```python
from build123d import *

# Parameters (mm, degrees)
SKETCH_1_R             = 11
EXTRUDE_1_DEPTH        = 32
HOLE_WIZARD_M2_1_D     = 1.6
HOLE_WIZARD_M2_1_DEPTH = 5.2
HOLE_WIZARD_M2_1_TIP   = 0.480688495
CUT_EXTRUDE_START      = -3
SKETCH_5_R             = 11.838448527
SKETCH_5_R_2           = 10.75
CUT_EXTRUDE_1_DEPTH    = 0.05
CUT_EXTRUDE_START_2    = -30
SKETCH_5_2_R           = 11.838448527
SKETCH_5_2_R_2         = 10.75
CUT_EXTRUDE_2_DEPTH    = 0.05
SKETCH_6_R             = 12
EXTRUDE_2_DEPTH        = 13
SKETCH_7_R             = 5
EXTRUDE_3_DEPTH        = 3
SKETCH_8_R             = 3
EXTRUDE_4_DEPTH        = 4
SKETCH_9_R             = 1.5
EXTRUDE_5_DEPTH        = 13
SKETCH_10_W            = 5.142844332
SKETCH_10_H            = 1.571012966
CUT_EXTRUDE_3_DEPTH    = 8
HOLE_WIZARD_M2_2_D     = 1.6
HOLE_WIZARD_M2_2_DEPTH = 5.2
HOLE_WIZARD_M2_2_TIP   = 0.480688495


with BuildPart() as part:
    # Sketch 1 → Extrude 1 (new body)
    with BuildSketch(Plane.XY):
        Circle(SKETCH_1_R)
    extrude(amount=EXTRUDE_1_DEPTH)

    # Hole Wizard M2 _1
    with Locations(Plane(origin=(0, 8.5, 32), x_dir=(1, 0, 0), z_dir=(0, 0, 1))):
        with Locations((0, 0), (0, -17)):
            Hole(HOLE_WIZARD_M2_1_D / 2, depth=HOLE_WIZARD_M2_1_DEPTH)
            with Locations((0, 0, -(HOLE_WIZARD_M2_1_DEPTH + HOLE_WIZARD_M2_1_TIP / 2))):  # 118° drill point
                Cone(0, HOLE_WIZARD_M2_1_D / 2, HOLE_WIZARD_M2_1_TIP, mode=Mode.SUBTRACT)

    # Sketch 5 → Cut-Extrude 1 (cut)
    with BuildSketch(Plane(origin=(0, 0, 0), x_dir=(-1, 0, 0), z_dir=(0, 0, -1)).offset(CUT_EXTRUDE_START)):
        Circle(SKETCH_5_R)
        Circle(SKETCH_5_R_2, mode=Mode.SUBTRACT)
    extrude(amount=-CUT_EXTRUDE_1_DEPTH, mode=Mode.SUBTRACT)

    # Sketch 5_2 → Cut-Extrude 2 (cut)
    with BuildSketch(Plane(origin=(0, 0, 0), x_dir=(-1, 0, 0), z_dir=(0, 0, -1)).offset(CUT_EXTRUDE_START_2)):
        Circle(SKETCH_5_2_R)
        Circle(SKETCH_5_2_R_2, mode=Mode.SUBTRACT)
    extrude(amount=-CUT_EXTRUDE_2_DEPTH, mode=Mode.SUBTRACT)

    # Sketch 6 → Extrude 2 (add)
    with BuildSketch(Plane.XY.offset(32)):
        with Locations(Location((0, 0, 0), (0, 0, 180))):
            Circle(SKETCH_6_R)
    extrude(amount=EXTRUDE_2_DEPTH)

    # Sketch 7 → Extrude 3 (add)
    with BuildSketch(Plane.XY.offset(45)):
        Circle(SKETCH_7_R)
    extrude(amount=EXTRUDE_3_DEPTH)

    # Sketch 8 → Extrude 4 (add)
    with BuildSketch(Plane.XY.offset(45)):
        Circle(SKETCH_8_R)
    extrude(amount=EXTRUDE_4_DEPTH)

    # Sketch 9 → Extrude 5 (add)
    with BuildSketch(Plane.XY.offset(45)):
        with Locations(Location((0, 0, 0), (0, 0, 180))):
            Circle(SKETCH_9_R)
    extrude(amount=EXTRUDE_5_DEPTH)

    # Sketch 10 → Cut-Extrude 3 (cut)
    with BuildSketch(Plane.XY.offset(58)):
        with Locations((0.334320666, 1.635506483)):
            Rectangle(SKETCH_10_W, SKETCH_10_H)
    extrude(amount=-CUT_EXTRUDE_3_DEPTH, mode=Mode.SUBTRACT)

    # Hole Wizard M2 _2
    with Locations(Plane(origin=(0, 9.8, 45), x_dir=(1, 0, 0), z_dir=(0, 0, 1))):
        with Locations((0, 0), (8.487048957, -14.7), (-8.487048957, -14.7)):
            Hole(HOLE_WIZARD_M2_2_D / 2, depth=HOLE_WIZARD_M2_2_DEPTH)
            with Locations((0, 0, -(HOLE_WIZARD_M2_2_DEPTH + HOLE_WIZARD_M2_2_TIP / 2))):  # 118° drill point
                Cone(0, HOLE_WIZARD_M2_2_D / 2, HOLE_WIZARD_M2_2_TIP, mode=Mode.SUBTRACT)


solid = part.part
```
Geometry check sheet. Reference: the model listing, model coordinates, mm. A direction names the side the tool comes from. Coordinates: 2 decimals unless noted, no trailing zeros. Order: outer loops, then holes, each group sorted by start corner. A loop starts at its lowest first (then second) coordinate and runs counter-clockwise, first axis right, second up. Notation, with made-up numbers: (22, 28.25) - (78, 28.25) arc R19 cw to (78, 41.25) - close; hole circle Ø7 at (4, 10). An arc over 180 degrees is marked (long way). Answer as a JSON object with one key per item and string values. Group by question number.
Item 1: Sectioned sample at A-A, the plane z = 29. Record the cut outline in (x, y).
Item 2: Tool access check on faces 5 (the face through (-2.38, -10.74, 1.48)), 6 (the face through (-0.1, -3.3, 48)), 7 (the face through (0.075, 8.617, 26.403)). Record the directions out of +Z, -Z, +X, -X, +Y, -Y that give a thin tool (end or side, any length) a straight path to the whole face; none if there is none.
Item 3: Sectioned sample at D-D, the plane x = -3.75. Record the cut outline in (y, z).
Item 4: Sectioned sample at C-C, the plane z = 54.5. Record the cut outline in (x, y).
Item 5: Draft check along X on faces 1 (the face through (-5.2, -0.2, 45)), 2 (the face through (0.104, 9.293, 29.364)), 3 (the face through (8.562, -4.783, 39.403)), 4 (the face through (-3, 0.1, 48.5)). Enter one of: +X half, -X half, draft (parallel to the pull), parting line (faces both ways), or undercut.
Item 6: Scan lines: probe 1 along Y at (x, z) = (0, 29.7); probe 2 along Y at (x, z) = (0, 43.6); probe 3 along Z at (x, y) = (10.25, 0.5). Record each from-to range of solid material in increasing order.
Item 7: Sectioned sample at B-B, the plane x = -10. Record the cut outline in (y, z), and give its area (3 significant figures).
Item 8: Depth check by flat-ended pin: pin 1 Ø10 at (y, z) = (1.5, 16.5) entering from +X; pin 2 Ø1.3 at (x, y) = (0, 8.5) entering from +Z; pin 3 Ø3 at (y, z) = (-9, 12) entering from +X. Enter the tip coordinate at first touch or a pass-through.
Resolved:
{
 "1": {"outline": "circle Ø22 at (0, 0); hole circle Ø1.6 at (0, -8.5); hole circle Ø1.6 at (0, 8.5)"},
 "2": {"face 5": "-Z", "face 6": "+Z", "face 7": "none"},
 "3": {"outline": "(-11.4, 32) - (-10.34, 32) - (-10.34, 30.05) - (-10.07, 30.05) - (-10.07, 30) - (-10.34, 30) - (-10.34, 3.05) - (-10.07, 3.05) - (-10.07, 3) - (-10.34, 3) - (-10.34, 0) - (10.34, 0) - (10.34, 3) - (10.07, 3) - (10.07, 3.05) - (10.34, 3.05) - (10.34, 30) - (10.07, 30) - (10.07, 30.05) - (10.34, 30.05) - (10.34, 32) - (11.4, 32) - (11.4, 45) - (3.31, 45) - (3.31, 48) - (-3.31, 48) - (-3.31, 45) - (-11.4, 45) - close"},
 "4": {"outline": "(-1.24, 0.85) arc R1.5 ccw (long way) to (1.24, 0.85) - close"},
 "5": {"face 1": "draft", "face 2": "undercut", "face 3": "undercut", "face 4": "parting line"},
 "6": {"probe 1": "-11 to -9.3, -7.7 to 7.7, 9.3 to 11", "probe 2": "-12 to 9, 10.6 to 12", "probe 3": "0 to 45"},
 "7": {"outline": "(-6.63, 32) - (-4.58, 32) - (-4.58, 30.05) - (-3.94, 30.05) - (-3.94, 30) - (-4.58, 30) - (-4.58, 3.05) - (-3.94, 3.05) - (-3.94, 3) - (-4.58, 3) - (-4.58, 0) - (4.58, 0) - (4.58, 3) - (3.94, 3) - (3.94, 3.05) - (4.58, 3.05) - (4.58, 30) - (3.94, 30) - (3.94, 30.05) - (4.58, 30.05) - (4.58, 32) - (6.63, 32) - (6.63, 45) - (-6.63, 45) - close", "area": "466 mm^2"},
 "8": {"pin 1": "x = 11", "pin 2": "z = 45", "pin 3": "x = 8.05"}
}
